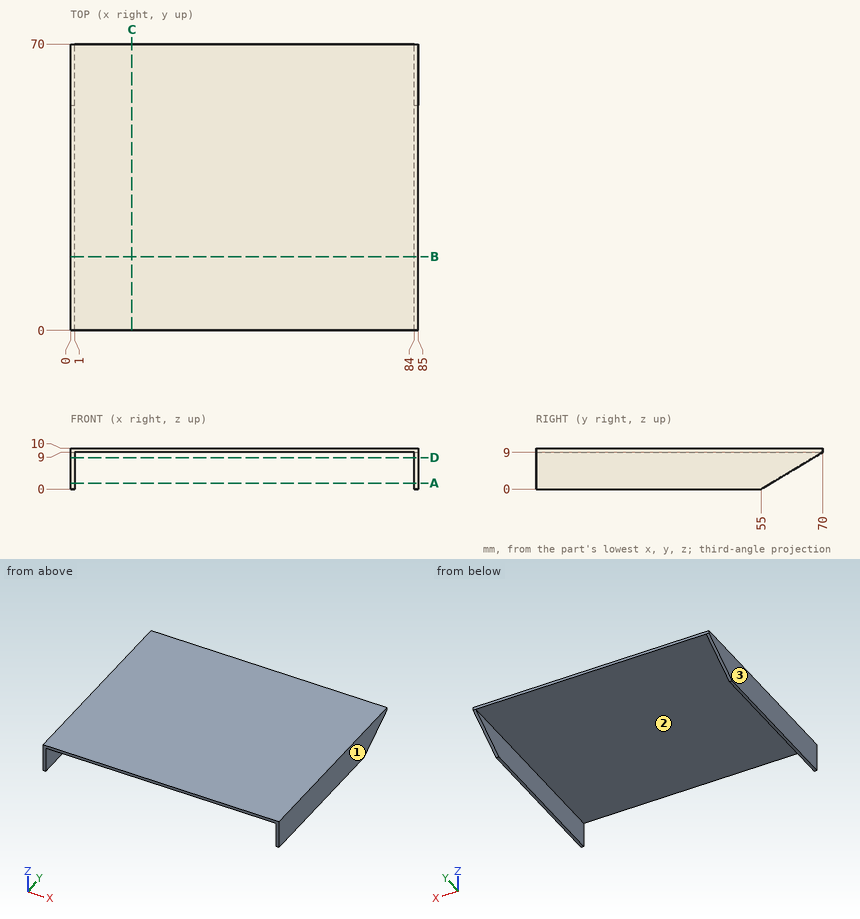
Geometry: see drawing. Coordinates: mm, zero at the bounding-box minimum. Coordinates: 2 decimals unless noted, no trailing zeros. Write each loop counter-clockwise with the first axis right and the second up, starting at its lowest first coordinate (ties: lowest second). Pieces come first, ordered by that corner, then holes.
1) Section C-C on x = 15. Output: boundary loops of the cut face in (y, z), and give its area (3 significant figures).
2) Material intervals for line 1 along X through (y, z) = (8, 2.5); line 2 along Z through (x, y) = (60, 18.5), sorted ascending.
3) Mould query, pull axis X, two halves, no side actions, for the marked faces 1, 2 and 3. Classes: pulls with the +X half, pulls with the -X half, needs draft (parallel to the pull), parting line crosses it, or undercut.
4) Section D-D on z = 7.75. Output: boundary loops of the cut face in (x, y), and give its area (3 significant figures).
5) Section B-B on y = 18. Output: boundary loops of the cut face in (x, z), and give its area (3 significant figures).
6) Pin query (flat end, axial travel): pin 1 Ø1 at (x, y) = (41, 45.5) entering from -Z. Return the tip coordinate at first contact, or that it passes through.
7) Section A-A on z = 1.5. Output: boundary loops of the cut face in (x, y), and give its area (3 significant figures).
Check result:
1. outline: (0, 9) - (70, 9) - (70, 10) - (0, 10) - close
1. area: 70.0 mm2
2. line 1: x = 0 to 1, 84 to 85
2. line 2: z = 9 to 10
3. face 1: pulls with the +X half
3. face 2: undercut
3. face 3: pulls with the -X half
4. outline: (0, 0) - (1, 0) - (1, 67.92) - (0, 67.92) - close; (84, 0) - (85, 0) - (85, 67.92) - (84, 67.92) - close
4. area: 136 mm2
5. outline: (0, 0) - (1, 0) - (1, 9) - (84, 9) - (84, 0) - (85, 0) - (85, 10) - (0, 10) - close
5. area: 103 mm2
6. pin 1: stops at z = 9
7. outline: (0, 0) - (1, 0) - (1, 57.5) - (0, 57.5) - close; (84, 0) - (85, 0) - (85, 57.5) - (84, 57.5) - close
7. area: 115 mm2
